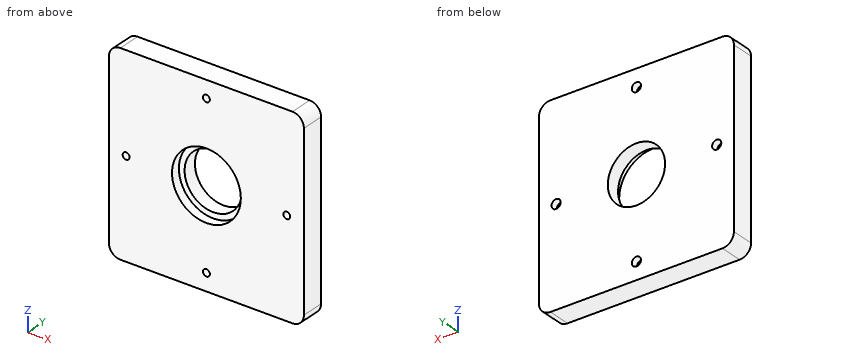
from build123d import *

# Parameters (mm, degrees)
SKETCH2_W                               = 170
SKETCH2_H                               = 170
BOSS_EXTRUDE1_DEPTH                     = 20
FILLET1_R                               = 10
FILLET2_R                               = 10
FILLET3_R                               = 10
FILLET4_R                               = 10
SKETCH11_R                              = 30
CUT_EXTRUDE3_DEPTH                      = 8
SKETCH16_R                              = 25
CUT_EXTRUDE4_DEPTH                      = 96
CBORE_FOR_M5_HEX_HEAD_BOLT4_D           = 6
CBORE_FOR_M5_HEX_HEAD_BOLT4_CBORE_D     = 8
CBORE_FOR_M5_HEX_HEAD_BOLT4_CBORE_DEPTH = 6


with BuildPart() as part:
    # Sketch2 → Boss-Extrude1 (new body)
    with BuildSketch(Plane(origin=(0, 0, 0), x_dir=(1, 0, 0), z_dir=(0, 1, 0))):
        Rectangle(SKETCH2_W, SKETCH2_H)
    extrude(amount=BOSS_EXTRUDE1_DEPTH)

    # Fillet1
    fillet1_edges = [part.edges().sort_by_distance(p)[0] for p in [
        (85, 10, 85),
    ]]
    fillet(fillet1_edges, radius=FILLET1_R)

    # Fillet2
    fillet2_edges = [part.edges().sort_by_distance(p)[0] for p in [
        (85, 10, -85),
    ]]
    fillet(fillet2_edges, radius=FILLET2_R)

    # Fillet3
    fillet3_edges = [part.edges().sort_by_distance(p)[0] for p in [
        (-85, 10, -85),
    ]]
    fillet(fillet3_edges, radius=FILLET3_R)

    # Fillet4
    fillet4_edges = [part.edges().sort_by_distance(p)[0] for p in [
        (-85, 10, 85),
    ]]
    fillet(fillet4_edges, radius=FILLET4_R)

    # Sketch11 → Cut-Extrude3 (cut)
    with BuildSketch(Plane.XZ):
        Circle(SKETCH11_R)
    extrude(amount=-CUT_EXTRUDE3_DEPTH, mode=Mode.SUBTRACT)

    # Sketch16 → Cut-Extrude4 (cut)
    with BuildSketch(Plane.XZ.offset(-8)):
        Circle(SKETCH16_R)
    extrude(amount=-CUT_EXTRUDE4_DEPTH, mode=Mode.SUBTRACT)

    # CBORE for M5 Hex Head Bolt4 (through all)
    with Locations(Plane(origin=(0, 20, 0), x_dir=(1, 0, 0), z_dir=(0, 1, 0))):
        with Locations((0, 70), (0, -70), (70, 0), (-70, 0)):
            CounterBoreHole(CBORE_FOR_M5_HEX_HEAD_BOLT4_D / 2, CBORE_FOR_M5_HEX_HEAD_BOLT4_CBORE_D / 2, CBORE_FOR_M5_HEX_HEAD_BOLT4_CBORE_DEPTH)


solid = part.part
For this review, take the finished solid that the model builds, in its own axes (mm). Give positions to 0.01 mm unless a question says otherwise; leave off trailing zeros. Loops run counter-clockwise (first coordinate to the right, second up) from the corner with the lowest first, then second, coordinate; pieces in that order, holes last. Notation, with made-up numbers: M 71,4.25 L 110,4.25 A30 ccw 110,35.25 Z; hole C 0.5,86 d9. An arc over 180 degrees is marked long. Put each result on its own line as item: value. Start each with the question number.
(1) Add section D-D, the plane x = -70. Write out the cut boundary in (y, z).
(2) Add section C-C, the plane z = 70. Write out the cut boundary in (x, y).
(3) Add section A-A, the plane x = 0. Write out the cut boundary in (y, z).
(4) For pin 1 (6.5 mm diameter, centred on x = 0, z = 70, fed in from -Y); pin 2 (7 mm diameter, centred on x = 70, z = 0, fed in from +Y); pin 3 (5 mm diameter, centred on x = 0, z = -70, fed in from -Y), all flat-tipped, find the tip position at first contact; note any pin that passes through.
(5) Wall thickness on L1, parallel to Z at x = 0, y = 14.75; L2, parallel to Z at x = -70, y = 4.75; L3, parallel to X at y = 17, z = 70: over which ranges is each line inside the solid? List them lowest first.
(6) Add section B-B, the plane y = 3.5. Write out the cut boundary in (x, z).
Result:
1. outline: M 0,-85 L 20,-85 L 20,-4 L 14,-4 L 14,-3 L 0,-3 Z; M 0,3 L 14,3 L 14,4 L 20,4 L 20,85 L 0,85 Z
2. outline: M -85,0 L -3,0 L -3,14 L -4,14 L -4,20 L -85,20 Z; M 3,0 L 85,0 L 85,20 L 4,20 L 4,14 L 3,14 Z
3. outline: M 0,-85 L 20,-85 L 20,-74 L 14,-74 L 14,-73 L 0,-73 Z; M 0,-67 L 14,-67 L 14,-66 L 20,-66 L 20,-25 L 8,-25 L 8,-30 L 0,-30 Z; M 0,30 L 8,30 L 8,25 L 20,25 L 20,66 L 14,66 L 14,67 L 0,67 Z; M 0,73 L 14,73 L 14,74 L 20,74 L 20,85 L 0,85 Z
4. pin 1: stops at y = 0
4. pin 2: stops at y = 14
4. pin 3: passes through
5. L1: z = -85 to -74, -66 to -25, 25 to 66, 74 to 85
5. L2: z = -85 to -3, 3 to 85
5. L3: x = -85 to -4, 4 to 85
6. outline: M -85,-75 A10 ccw -75,-85 L 75,-85 A10 ccw 85,-75 L 85,75 A10 ccw 75,85 L -75,85 A10 ccw -85,75 Z; hole C -70,0 d6; hole C 0,0 d60; hole C 0,-70 d6; hole C 0,70 d6; hole C 70,0 d6
